Verification items for the finished model (mm, model axes). A direction names the side the tool comes from. Coordinates: 2 decimals unless noted, no trailing zeros. Write each loop counter-clockwise with the first axis right and the second up, starting at its lowest first coordinate (ties: lowest second). Pieces come first, ordered by that corner, then holes. Notation, with made-up numbers: M 89.25,38 L 103.25,38 A5 ccw 103.25,47 Z; hole C 21,57 d3. An arc over 180 degrees is marked long. One line per item, written item: value.
```python
from build123d import *

# Parameters (mm, degrees)
SKETCH1_W          = 15
SKETCH1_H          = 4
CHAMFER1_SIZE      = 0.4
SKETCH2_W          = 23
SKETCH2_H          = 3
TAPPED_HOLE1_D     = 2.5
TAPPED_HOLE1_DEPTH = 8.5
TAPPED_HOLE1_TIP   = 0.751075774
TAPPED_HOLE2_D     = 2.5
TAPPED_HOLE2_DEPTH = 8.5
TAPPED_HOLE2_TIP   = 0.751075774
CHAMFER2_SIZE      = 0.4
CHAMFER3_SIZE      = 0.4


with BuildPart() as part:
    # Sketch1 → Revolve1 (revolve)
    with BuildSketch(Plane.XY):
        with Locations((7.5, 2)):
            Rectangle(SKETCH1_W, SKETCH1_H)
    revolve(axis=Axis((15, 0, 0), (-1, 0, 0)))

    # Chamfer1
    chamfer1_edges = [part.edges().sort_by_distance(p)[0] for p in [
        (15, -4, 0),
        (0, -4, 0),
    ]]
    chamfer(chamfer1_edges, length=CHAMFER1_SIZE)

    # Sketch2 → Revolve2 (revolve)
    with BuildSketch(Plane.XY, mode=Mode.PRIVATE) as revolve2_sk:
        with Locations((7.5, 1.5)):
            Rectangle(SKETCH2_W, SKETCH2_H)
    revolve(revolve2_sk.sketch.rotate(Axis((-4, 0, 0), (1, 0, 0)), 90), axis=Axis((-4, 0, 0), (1, 0, 0)))

    # Tapped Hole1
    with Locations(Plane(origin=(-4, 0, 0), x_dir=(0, 0, -1), z_dir=(-1, 0, 0))):
        with Locations((0, 0)):
            Hole(TAPPED_HOLE1_D / 2, depth=TAPPED_HOLE1_DEPTH)
            with Locations((0, 0, -(TAPPED_HOLE1_DEPTH + TAPPED_HOLE1_TIP / 2))):  # 118° drill point
                Cone(0, TAPPED_HOLE1_D / 2, TAPPED_HOLE1_TIP, mode=Mode.SUBTRACT)

    # Tapped Hole2
    with Locations(Plane(origin=(19, 1.854743126, 0.460903034), x_dir=(0, 0, -1), z_dir=(1, 0, 0))):
        with Locations((0.460903034, -1.854743126)):
            Hole(TAPPED_HOLE2_D / 2, depth=TAPPED_HOLE2_DEPTH)
            with Locations((0, 0, -(TAPPED_HOLE2_DEPTH + TAPPED_HOLE2_TIP / 2))):  # 118° drill point
                Cone(0, TAPPED_HOLE2_D / 2, TAPPED_HOLE2_TIP, mode=Mode.SUBTRACT)

    # Chamfer2
    chamfer2_edges = [part.edges().sort_by_distance(p)[0] for p in [
        (-4, 0, -3),
    ]]
    chamfer(chamfer2_edges, length=CHAMFER2_SIZE)

    # Chamfer3
    chamfer3_edges = [part.edges().sort_by_distance(p)[0] for p in [
        (19, 0, -3),
    ]]
    chamfer(chamfer3_edges, length=CHAMFER3_SIZE)


solid = part.part
```
Item 1: Cross-section at B-B, the plane x = 1.25. Enter the section's corners in (y, z), and give its area (3 significant figures).
The answers:
outline: C 0,0 d8; hole C 0,0 d2.5
area: 45.4 mm²
Item 2: Go/stop test with flat-tipped pins: P1, Ø1, axis at x = 6.5, y = 3, coming from the -Z side; P2, Ø3, axis at x = 15.5, y = -3, coming from the +Z side; P3, Ø1.5, axis at y = 0, z = 0, coming from the -X side. Record where each tip stops, or that it passes through.
The answers:
P1: stops at z = -3.12
P2: stops at z = 3.57
P3: stops at x = 4.8
Item 3: Cross-section at A-A, the plane x = 17.25. Enter the section's corners in (y, z).
The answers:
outline: C 0,0 d6; hole C 0,0 d2.5
Item 4: Draft check along Y on faces 4 (the face through (19, 1, 1)), 5 (the face through (-1.77, -0.9, 2.86)), 6 (the face through (5.12, 0.21, 0.05)). Enter one of: released by +Y, released by -Y, zero draft, split by the parting line, or undercut.
The answers:
face 4: zero draft
face 5: split by the parting line
face 6: undercut
Item 5: Scan lines: line 1 (Y direction, x = 1.25, z = 0); line 2 (X direction, y = 2.75, z = -1.5); line 3 (Z direction, x = 0.75, y = -0.5). Record each from-to range of solid material in increasing order.
The answers:
line 1: y = -4 to -1.25, 1.25 to 4
line 2: x = 0 to 15
line 3: z = -3.97 to -1.15, 1.15 to 3.97
Item 6: Access from +Z, -Z, +X, -X, +Y, -Y to the whole of each face (thin tool, end or side, straight path). Record for faces 1 (the face through (-4, 1, 1)), 2 (the face through (15, 1, -3)), 3 (the face through (0.31, 1.22, -0.27)).
The answers:
face 1: +Z, -Z, -X, +Y, -Y
face 2: +X
face 3: -X
